```python
from build123d import *

# Parameters (mm, degrees)
SKETCH1_R           = 16.51
BOSS_EXTRUDE1_DEPTH = 44.831
SKETCH2_R           = 9.398
CUT_EXTRUDE1_DEPTH  = 51.546797732
SKETCH3_R           = 10.16
CUT_EXTRUDE2_DEPTH  = 4.953
SKETCH4_R           = 1.7272
CUT_EXTRUDE3_DEPTH  = 12.7
CIRPATTERN1_COUNT   = 4
CUT_EXTRUDE4_START  = -0.381
SKETCH5_R           = 10.16
CUT_EXTRUDE4_DEPTH  = 0.381
SKETCH7_W           = 9.037015708
SKETCH7_H           = 32.512
SKETCH9_R           = 1.7526
CUT_EXTRUDE6_DEPTH  = 10.16
CIRPATTERN3_COUNT   = 6
CUT_EXTRUDE7_DEPTH  = 15.24
CIRPATTERN4_COUNT   = 6
CUT_EXTRUDE8_START  = -2.54
SKETCH13_R          = 16.51
CUT_EXTRUDE8_DEPTH  = 2.54


with BuildPart() as part:
    # Sketch1 → Boss-Extrude1 (new body)
    with BuildSketch(Plane(origin=(0, 0, 0), x_dir=(1, 0, 0), z_dir=(0, 1, 0))):
        with Locations(Location((0, 0, 0), (0, 0, 90))):
            Circle(SKETCH1_R)
    extrude(amount=BOSS_EXTRUDE1_DEPTH)

    # Sketch2 → Cut-Extrude1 (cut, through all)
    with BuildSketch(Plane(origin=(0, 44.831, 0), x_dir=(1, 0, 0), z_dir=(0, 1, 0))):
        with Locations(Location((0, 0, 0), (0, 0, 270))):
            Circle(SKETCH2_R)
    extrude(amount=-CUT_EXTRUDE1_DEPTH, mode=Mode.SUBTRACT)

    # Sketch3 → Cut-Extrude2 (cut)
    with BuildSketch(Plane(origin=(0, 44.831, 0), x_dir=(1, 0, 0), z_dir=(0, 1, 0))):
        with Locations(Location((0, 0, 0), (0, 0, 270))):
            Circle(SKETCH3_R)
    extrude(amount=-CUT_EXTRUDE2_DEPTH, mode=Mode.SUBTRACT)

    # Sketch4 → Cut-Extrude3 (cut)
    with BuildSketch(Plane(origin=(0, 44.831, 0), x_dir=(1, 0, 0), z_dir=(0, 1, 0))):
        with Locations(Location((-12.7, 0, 0), (0, 0, 270))):
            Circle(SKETCH4_R)
    cut_extrude3 = extrude(amount=-CUT_EXTRUDE3_DEPTH, mode=Mode.SUBTRACT)

    # CirPattern1: Cut-Extrude3 ×4 about axis
    cirpattern1_axis = Axis((0, 0, 0), (0, 1, 0))
    for i in range(1, CIRPATTERN1_COUNT):
        add(cut_extrude3.rotate(cirpattern1_axis, i * 360 / CIRPATTERN1_COUNT), mode=Mode.SUBTRACT)

    # Sketch5 → Cut-Extrude4 (cut)
    with BuildSketch(Plane.XZ.offset(CUT_EXTRUDE4_START)):
        with Locations(Location((0, 0, 0), (0, 0, 90))):
            Circle(SKETCH5_R)
    extrude(amount=CUT_EXTRUDE4_DEPTH, mode=Mode.SUBTRACT)

    # Sketch7 → Cut-Revolve2 (revolve, cut)
    with BuildSketch(Plane.XY, mode=Mode.PRIVATE) as cut_revolve2_sk:
        with Locations((-14.678507762, 21.336)):
            Rectangle(SKETCH7_W, SKETCH7_H)
    cut_revolve2 = revolve(cut_revolve2_sk.sketch.rotate(Axis((0, 0, 0), (0, 1, 0)), 270), axis=Axis((0, 0, 0), (0, 1, 0)), mode=Mode.SUBTRACT)

    # Sketch9 → Cut-Extrude6 (cut)
    with BuildSketch(Plane.XZ):
        with Locations(Location((0, -13.208, 0), (0, 0, 270))):
            Circle(SKETCH9_R)
    cut_extrude6 = extrude(amount=-CUT_EXTRUDE6_DEPTH, mode=Mode.SUBTRACT)

    # CirPattern3: Cut-Extrude6 ×6 about axis
    cirpattern3_axis = Axis((0, 0, 0), (0, 1, 0))
    for i in range(1, CIRPATTERN3_COUNT):
        add(cut_extrude6.rotate(cirpattern3_axis, i * 360 / CIRPATTERN3_COUNT), mode=Mode.SUBTRACT)

    # Sketch12 → Cut-Extrude7 (cut)
    with BuildSketch(Plane.XY.offset(16.51)):
        with BuildLine():
            Line((2.780051948, 32.164471738), (2.780051948, 9.304471738))
            ThreePointArc((2.780051948, 9.304471738), (0, 6.52441979), (-2.780051948, 9.304471738))
            Line((-2.780051948, 9.304471738), (-2.780051948, 32.164471738))
            ThreePointArc((-2.780051948, 32.164471738), (0, 34.944523686), (2.780051948, 32.164471738))
        make_face()
    cut_extrude7 = extrude(amount=-CUT_EXTRUDE7_DEPTH, mode=Mode.SUBTRACT)

    # CirPattern4: Cut-Revolve2, Cut-Extrude7 ×6 about axis
    cirpattern4_axis = Axis((0, 0, 0), (0, 1, 0))
    add([cut_revolve2.rotate(cirpattern4_axis, i * 360 / CIRPATTERN4_COUNT) for i in range(1, CIRPATTERN4_COUNT)], mode=Mode.SUBTRACT)
    add([cut_extrude7.rotate(cirpattern4_axis, i * 360 / CIRPATTERN4_COUNT) for i in range(1, CIRPATTERN4_COUNT)], mode=Mode.SUBTRACT)

    # Sketch13 → Cut-Extrude8 (cut)
    with BuildSketch(Plane(origin=(0, 44.831, 0), x_dir=(1, 0, 0), z_dir=(0, 1, 0)).offset(CUT_EXTRUDE8_START)):
        with Locations(Location((0, 0, 0), (0, 0, 90))):
            Circle(SKETCH13_R)
    extrude(amount=CUT_EXTRUDE8_DEPTH, mode=Mode.SUBTRACT)


solid = part.part
```
Input: part model. Units: mm. Frame: model coordinates. A direction names the side the tool comes from. Give positions to 0.01 mm unless a question says otherwise; leave off trailing zeros. Order: outer loops, then holes, each group sorted by start corner. A loop starts at its lowest first (then second) coordinate and runs counter-clockwise, first axis right, second up.
1. Cut plane B-B (y = 27.5). Return loops of the section in (x, z), and give its area (3 significant figures).
Computed:
outline: (-9.85, -2.48) - (-9.16, -2.08) arc R9.4 cw to (-9.16, 2.08) - (-9.85, 2.48) arc R10.16 ccw to start; (-7.07, -7.29) arc R10.16 ccw to (-2.78, -9.77) - (-2.78, -8.98) arc R9.4 cw to (-6.38, -6.9) - close; (-7.07, 7.29) - (-6.38, 6.9) arc R9.4 cw to (-2.78, 8.98) - (-2.78, 9.77) arc R10.16 ccw to start; (2.78, -9.77) arc R10.16 ccw to (7.07, -7.29) - (6.38, -6.9) arc R9.4 cw to (2.78, -8.98) - close; (2.78, 8.98) arc R9.4 cw to (6.38, 6.9) - (7.07, 7.29) arc R10.16 ccw to (2.78, 9.77) - close; (9.16, -2.08) - (9.85, -2.48) arc R10.16 ccw to (9.85, 2.48) - (9.16, 2.08) arc R9.4 cw to start
area: 21.0 mm2
2. Line query: probe 1 along X at (y, z) = (38.85, 0); probe 2 along Y at (x, z) = (-6, 11); probe 3 along Z at (x, y) = (-1, 2.5). Output: solid intervals per line, ascending.
Computed:
probe 1: x = -16.51 to -14.43, -10.97 to -9.4, 9.4 to 10.97, 14.43 to 16.51
probe 2: y = 0 to 5.08, 37.59 to 42.29
probe 3: z = -16.48 to -14.65, -11.77 to -9.34, 9.34 to 11.77, 14.65 to 16.48
3. Cut plane A-A (z = 0). State how many separate pieces and enclosed holes the cut face has, and give its area (3 significant figures).
Computed:
separate pieces: 4
enclosed holes: 0
area: 152 mm2
4. Pin query (flat end, axial travel): pin 1 Ø2 at (x, z) = (0, 13.208) entering from -Y; pin 2 Ø12 at (y, z) = (5.5, 2) entering from +X; pin 3 Ø2 at (x, y) = (-3, 11.5) entering from +Z; pin 4 Ø3 at (y, z) = (19.5, 10.5) entering from +X. Return the tip coordinate at first contact, or that it passes through.
Computed:
pin 1: passes through
pin 2: stops at x = 16.51
pin 3: stops at z = 9.77
pin 4: stops at x = 4.71
5. Set-up query: faces 1 (the face through (9.7, 2.5, -6.83)), 2 (the face through (10.987, 39.974, 0.225)), 3 (the face through (0.061, 34.944, -9.577)), 4 (the face through (-8.326, 34.944, 4.736)). Return all of +Z, -Z, +X, -X, +Y, -Y with unobstructed straight access to the full face (end or side cutting, diameter ignored); none if empty.
Computed:
face 1: -Y
face 2: +Y
face 3: +Z, -Z
face 4: none
6. Draft query along X for faces 5 (the face through (9.92, 21.56, 2.2)), 6 (the face through (10.8, 37.592, 0.2)), 7 (the face through (0.671, 2.504, 14.827)). Return one class per face: released by +X, released by -X, zero draft, split by the parting line, or undercut.
Computed:
face 5: split by the parting line
face 6: zero draft
face 7: undercut
7. Cut plane C-C (x = 5.5). Return loops of the section in (y, z), and give its area (3 significant figures).
Computed:
outline: (0, -15.57) - (5.08, -15.57) - (5.08, -8.54) - (37.59, -8.54) - (37.59, -15.57) - (42.29, -15.57) - (42.29, -8.54) - (39.88, -8.54) - (39.88, -7.62) - (0.38, -7.62) - (0.38, -8.54) - (0, -8.54) - close; (0, 8.54) - (0.38, 8.54) - (0.38, 7.62) - (39.88, 7.62) - (39.88, 8.54) - (42.29, 8.54) - (42.29, 15.57) - (37.59, 15.57) - (37.59, 8.54) - (5.08, 8.54) - (5.08, 15.57) - (0, 15.57) - close
area: 210 mm2
